from build123d import *

# Parameters (mm, degrees)
F1_DEPTH = 6.35


# Not quite as in the source:
# - a length typed as a fraction of an inch, garbled in the dataset ("3 / 203.2 mm" for 3/8 in), is restored


with BuildPart() as f1:
    # F0 (on Front) → F1 (new body)
    with BuildSketch(Plane.XZ):
        Polygon((-25.4000015863, 18.4), (-25.4, 16.4), (-19.05, 16.4), (-19.05, 0), (0, 0), (0, 2), (-17.05, 2), (-17.05, 40), (0, 40), (0, 42), (-19.05, 42), (-19.05, 18.4), align=None)
    extrude(amount=F1_DEPTH)

    # F2: F1 across plane


with BuildPart() as f1_1:
    add(f1.part)
    add(f1.part.mirror(Plane.YZ))


solid = f1_1.part
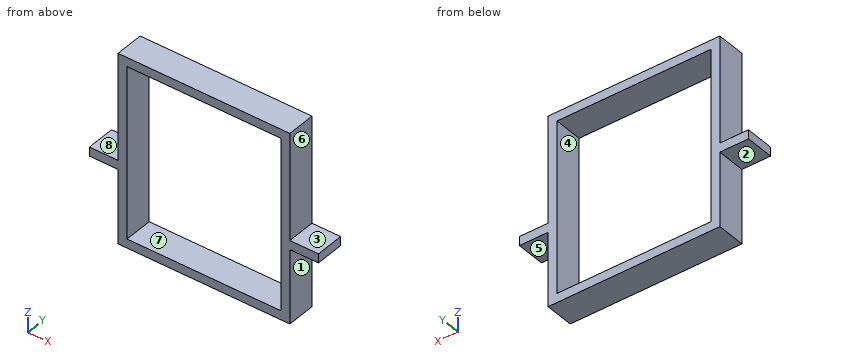
Source: CAD feature listing. Evaluate the final solid. Frame: model axes, mm. Face numbers are marked on the shaded views. A direction names the side the tool comes from. Coordinates: 2 decimals unless noted, no trailing zeros. Order: outer loops, then holes, each group sorted by start corner. A loop starts at its lowest first (then second) coordinate and runs counter-clockwise, first axis right, second up.
Item 1: Material intervals for line 1 (Z direction, x = 1, y = -0.75); line 2 (X direction, y = -1.75, z = 38); line 3 (X direction, y = -5.5, z = 18), sorted ascending.
Output values:
line 1: z = 0 to 2, 40 to 42
line 2: x = -19.05 to -17.05, 17.05 to 19.05
line 3: x = -25.4 to -17.05, 17.05 to 25.4
Item 2: Cut plane B-B (y = -3.5). Return loops of the section in (x, z), plus the area to 3 significant figures.
Output values:
outline: (-25.4, 16.4) - (-19.05, 16.4) - (-19.05, 0) - (19.05, 0) - (19.05, 16.4) - (25.4, 16.4) - (25.4, 18.4) - (19.05, 18.4) - (19.05, 42) - (-19.05, 42) - (-19.05, 18.4) - (-25.4, 18.4) - close; hole (-17.05, 2) - (17.05, 2) - (17.05, 40) - (-17.05, 40) - close
area: 330 mm2
Item 3: Pull-direction query (Z, two-part tool) for the marked faces 1, 2, 3 and 4; classes: pulls with the +Z half, pulls with the -Z half, needs draft (parallel to the pull), parting line crosses it, or undercut.
Output values:
face 1: needs draft
face 2: pulls with the -Z half
face 3: pulls with the +Z half
face 4: undercut
Item 4: Cut plane A-A (x = 11). Return loops of the section in (y, z), plus the area to 3 significant figures.
Output values:
outline: (-6.35, 0) - (0, 0) - (0, 2) - (-6.35, 2) - close; (-6.35, 40) - (0, 40) - (0, 42) - (-6.35, 42) - close
area: 25.4 mm2
Item 5: Cut plane C-C (z = 11.5). Return loops of the section in (x, y), plus the area to 3 significant figures.
Output values:
outline: (-19.05, -6.35) - (-17.05, -6.35) - (-17.05, 0) - (-19.05, 0) - close; (17.05, -6.35) - (19.05, -6.35) - (19.05, 0) - (17.05, 0) - close
area: 25.4 mm2
Item 6: Cut plane D-D (x = -20). Return loops of the section in (y, z), plus the area to 3 significant figures.
Output values:
outline: (-6.35, 16.4) - (0, 16.4) - (0, 18.4) - (-6.35, 18.4) - close
area: 12.7 mm2
Item 7: Set-up query: the marked faces 5, 6, 7 and 8. Return all of +Z, -Z, +X, -X, +Y, -Y with unobstructed straight access to the full face (end or side cutting, diameter ignored); none if empty.
Output values:
face 5: -Z, +X, +Y, -Y
face 6: +Z, +X, +Y, -Y
face 7: +Y, -Y
face 8: +Z, -X, +Y, -Y
Item 8: First-contact query: P1, Ø1.5, axis at y = -3, z = 19, coming from the +X side; P2, Ø1, axis at y = -3.5, z = 32, coming from the -X side; P3, Ø6, axis at x = -2, z = 35, coming from the +Y side; P4, Ø3, axis at x = 23, y = -1.5, coming from the +Z side. Flat tips, straight axial feed; report the tip coordinate or a pass-through.
Output values:
P1: stops at x = 25.4
P2: stops at x = -19.05
P3: passes through
P4: stops at z = 18.4
